Build history of the part. All positions in model axes, mm. A direction names the side the tool comes from. Give positions to 0.01 mm unless a question says otherwise; leave off trailing zeros. Order: outer loops, then holes, each group sorted by start corner. A loop starts at its lowest first (then second) coordinate and runs counter-clockwise, first axis right, second up. Notation, with made-up numbers: (51.5, 25.5) -> (88.5, 25.5) arc R14 cw to (88.5, 30.5) -> close; hole circle Ø5 at (88, 29). An arc over 180 degrees is marked (long way). One line per question, with ' | ' between items. Start each with the question number.
(1) Cut at B-B (y = -3). Give the cut face in (x, z).
(2) Pin check, flat tips, straight feed: pin 1 Ø6 at (x, z) = (6, 18) entering from -Y; pin 2 Ø10 at (x, z) = (10, 38.25) entering from +Y (3 decimals); pin 3 Ø5 at (x, z) = (10, -38.25) entering from +Y. Stop position of each tip, or through.
(3) Pull direction X, two halves, no side cores. Call faces 1 (the face through (10, -49.098, 38)), 2 (the face through (20, -8, -1)), 3 (the face through (10.04, -17.92, 43.79)): +X half, -X half, draft (parallel to the pull), parting line (faces both ways), or undercut.
(4) Drill centre lines: L1, parallel to Z at x = 10, y = -38.5; L2, parallel to Z at x = 12, y = -7; L3, parallel to X at y = -9, z = -38.25. Where is each one in solid material? Low to high. Write a range as from..to.
(5) Cut at A-A (y = -45). Give the cut face in (x, z).
(6) Cut at D-D (y = -34). Give the cut face in (x, z).
(7) Which spindle directions (+Z, -Z, +X, -X, +Y, -Y) get a long thin tool onto all of the face, cutting with end or side? Do faces 4 (the face through (9.56, -36.84, -45.72)), 5 (the face through (10.553, -14.325, 34.036)), 6 (the face through (5, -49.098, -42)). Say none if no direction does.
(8) Cut at C-C (x = 18.5). Give the cut face in (y, z).
from build123d import *

# Parameters (mm, degrees)
BOSS_EXTRUDE1_DEPTH          = 20
M8_TAPPED_HOLE1_D            = 6.8
M8_TAPPED_HOLE1_DEPTH        = 30
M8_TAPPED_HOLE1_CSINK_D      = 8.05
M8_TAPPED_HOLE1_CSINK_ANGLE  = 90
M8_TAPPED_HOLE1_TIP          = 2.042926105
M10_TAPPED_HOLE1_D           = 8.5
M10_TAPPED_HOLE1_DEPTH       = 27.5
M10_TAPPED_HOLE1_CSINK_D     = 10.05
M10_TAPPED_HOLE1_CSINK_ANGLE = 90
M10_TAPPED_HOLE1_TIP         = 2.553657631


with BuildPart() as part:
    # Sketch1 → Boss-Extrude1 (new body)
    with BuildSketch(Plane(origin=(0, 0, 0), x_dir=(0, 0, -1), z_dir=(1, 0, 0))):
        with BuildLine():
            Line((-48.35, 0), (48.35, 0))
            Line((48.35, 0), (48.35, -49.098))
            Line((48.35, -49.098), (36.35, -49.098))
            ThreePointArc((36.35, -49.098), (0, -12.748), (-36.35, -49.098))
            Line((-36.35, -49.098), (-48.35, -49.098))
            Line((-48.35, -49.098), (-48.35, 0))
        make_face()
    extrude(amount=BOSS_EXTRUDE1_DEPTH)

    # M8 Tapped Hole1
    with Locations(Plane(origin=(0, -49.098, 0), x_dir=(-1, 0, 0), z_dir=(0, -1, 0))):
        with Locations((-10, -42.35), (-10, 42.35)):
            CounterSinkHole(M8_TAPPED_HOLE1_D / 2, M8_TAPPED_HOLE1_CSINK_D / 2, depth=M8_TAPPED_HOLE1_DEPTH, counter_sink_angle=M8_TAPPED_HOLE1_CSINK_ANGLE)
            with Locations((0, 0, -(M8_TAPPED_HOLE1_DEPTH + M8_TAPPED_HOLE1_TIP / 2))):  # 118° drill point
                Cone(0, M8_TAPPED_HOLE1_D / 2, M8_TAPPED_HOLE1_TIP, mode=Mode.SUBTRACT)

    # M10 Tapped Hole1
    with Locations(Plane(origin=(0, 0, 0), x_dir=(1, 0, 0), z_dir=(0, 1, 0))):
        with Locations((10, -38.25), (10, 38.25)):
            CounterSinkHole(M10_TAPPED_HOLE1_D / 2, M10_TAPPED_HOLE1_CSINK_D / 2, depth=M10_TAPPED_HOLE1_DEPTH, counter_sink_angle=M10_TAPPED_HOLE1_CSINK_ANGLE)
            with Locations((0, 0, -(M10_TAPPED_HOLE1_DEPTH + M10_TAPPED_HOLE1_TIP / 2))):  # 118° drill point
                Cone(0, M10_TAPPED_HOLE1_D / 2, M10_TAPPED_HOLE1_TIP, mode=Mode.SUBTRACT)


solid = part.part
Result set:
1) outline: (0, -48.35) -> (20, -48.35) -> (20, 48.35) -> (0, 48.35) -> close; hole circle Ø8.5 at (10, -38.25); hole circle Ø8.5 at (10, 38.25)
2) pin 1: stops at y = -19.43 | pin 2: stops at y = -0.025 | pin 3: stops at y = -28.55
3) face 1: draft | face 2: +X half | face 3: undercut
4) L1: z = -48.35..-45.75, -38.95..-34.77, 34.77..38.95, 45.75..48.35 | L2: z = -48.35..-42, -34.5..34.5, 42..48.35 | L3: x = 0..5.75, 14.25..20
5) outline: (0, -48.35) -> (20, -48.35) -> (20, -36.12) -> (0, -36.12) -> close; (0, 36.12) -> (20, 36.12) -> (20, 48.35) -> (0, 48.35) -> close; hole circle Ø6.8 at (10, -42.35); hole circle Ø6.8 at (10, 42.35)
6) outline: (0, -48.35) -> (20, -48.35) -> (20, -33.07) -> (0, -33.07) -> close; (0, 33.07) -> (20, 33.07) -> (20, 48.35) -> (0, 48.35) -> close; hole circle Ø6.8 at (10, -42.35); hole circle Ø6.8 at (10, 42.35)
7) face 4: -Y | face 5: +Y | face 6: +Z, -Z, +X, -X, -Y
8) outline: (-49.1, -48.35) -> (0, -48.35) -> (0, 48.35) -> (-49.1, 48.35) -> (-49.1, 36.35) arc R36.35 cw to (-49.1, -36.35) -> close
